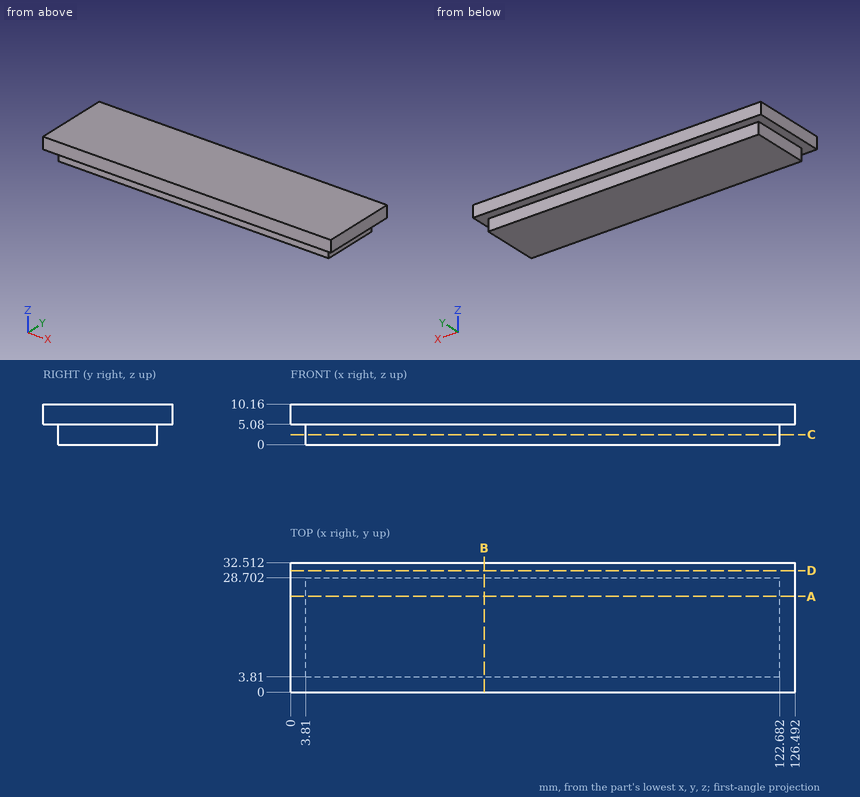
Part print with two shaded views. Sizes in mm from the minimum x, y, z corner. Round coordinates to 2 decimals unless told otherwise and drop trailing zeros. Loops run counter-clockwise (first coordinate to the right, second up) from the corner with the lowest first, then second, coordinate; pieces in that order, holes last. Notation, with made-up numbers: (-4, 79) - (8, 79) arc R33 ccw to (8, 108) - close; hole circle Ø6 at (78.25, 83). An arc over 180 degrees is marked (long way). Put each result on its own line as item: value.
1. Slice it at D-D on y = 30.5. List the corners of the cut face in (x, z), and give its area (3 significant figures).
Geometry check:
outline: (0, 5.08) - (126.49, 5.08) - (126.49, 10.16) - (0, 10.16) - close
area: 643 mm²
2. Slice it at C-C on z = 2.5. List the corners of the cut face in (x, y).
Geometry check:
outline: (3.81, 3.81) - (122.68, 3.81) - (122.68, 28.7) - (3.81, 28.7) - close
3. Slice it at B-B on x = 48.5. List the corners of the cut face in (y, z), and give its area (3 significant figures).
Geometry check:
outline: (0, 5.08) - (3.81, 5.08) - (3.81, 0) - (28.7, 0) - (28.7, 5.08) - (32.51, 5.08) - (32.51, 10.16) - (0, 10.16) - close
area: 292 mm²
4. Slice it at A-A on y = 24. List the corners of the cut face in (x, z).
Geometry check:
outline: (0, 5.08) - (3.81, 5.08) - (3.81, 0) - (122.68, 0) - (122.68, 5.08) - (126.49, 5.08) - (126.49, 10.16) - (0, 10.16) - close
5. Wall check: line 1 (Y direction, x = 49.5, z = 4.25); line 2 (X direction, y = 16, z = 1); line 3 (Z direction, x = 92, y = 1). Give the ranges that are in metal, low to high.
Geometry check:
line 1: 3.81 to 28.7
line 2: 3.81 to 122.68
line 3: 5.08 to 10.16
6. Pin check, flat tips, straight feed: P1, Ø2, axis at x = 64.5, z = 3, coming from the -Y side; P2, Ø1.5, axis at x = 61, z = 2.5, coming from the +Y side; P3, Ø5.5, axis at y = 15, z = 2, coming from the -X side. Stop position of each tip, or through.
Geometry check:
P1: y = 3.81
P2: y = 28.7
P3: x = 3.81
